The listing builds one solid part. Answer for the finished solid, in the listing's coordinates (mm). A direction names the side the tool comes from. Give positions to 0.01 mm unless a question says otherwise; leave off trailing zeros. Write each loop counter-clockwise with the first axis right and the second up, starting at its lowest first coordinate (ties: lowest second). Pieces come first, ordered by that corner, then holes. Notation, with made-up numbers: (78.25, -21) -> (89.25, -21) arc R25 ccw to (89.25, 17) -> close; hole circle Ø6 at (-3, -3). An arc over 180 degrees is marked (long way). Put each result on its own line as item: value. Start each with the question number.
1) For faces 1 (the flat face through (76.2, -8, 13)), 2 (the flat face through (-82.55, -8, 165)), 3 (the cylindrical face through (79.44, 20.35, 88.01)), determine the directions among +Z, -Z, +X, -X, +Y, -Y from which every point of the face is accessible in a straight line to the end or side of a thin tool.
2) Flat-ended cylindrical pins translate along their axes: pin 1 Ø2.5 at (y, z) = (-29.82, 158.75) entering from +X; pin 2 Ø1.9 at (x, y) = (-80, -18.5) entering from -Z; pin 3 Ø2 at (x, z) = (37, 61.5) entering from -Y; pin 4 Ø2 at (x, z) = (57.5, 140) entering from +Y. Find the tip coordinate at first contact, or state that the pin passes through.
3) A cutting plane is placed at C-C (x = 0). Write down the section's boundary in (y, z).
4) A cutting plane is placed at D-D (z = 92). Write down the section's boundary in (x, y) (3 decimals).
5) A cutting plane is placed at B-B (y = 80.5). Write down the section's boundary in (x, z).
6) A cutting plane is placed at A-A (y = -1.5). Write down the section's boundary in (x, z).
7) For a pull along X with two mould halves and no side action, classify faces 4 (the flat face through (-79, -39.977, 13)), 5 (the flat face through (-82.55, -8, 13)), 6 (the flat face through (-76.2, -8, 165)), 7 (the cylindrical face through (1.676, 99.704, 87.655)) as released by +X, released by -X, zero draft, split by the parting line, or undercut.
8) Find the intervals of material crossed by line 1 along X through (y, z) = (13.5, 159.5); line 2 along X through (y, z) = (84.5, 110); line 3 along Y through (x, z) = (-35, 93.5), in increasing order. Write a range as from..to.
from build123d import *

# Parameters (mm, degrees)
EXTRUDE_THIN1_DEPTH     = 177.8
SKETCH7_W               = 6.35
SKETCH7_H               = 25.4
BOSS_EXTRUDE2_DEPTH     = 63.5
SKETCH11_R              = 2
CUT_EXTRUDE1_DEPTH      = 6.35
MIRROR2_COPY_1_SKETCH_W = 6.35
MIRROR2_COPY_1_SKETCH_H = 25.4
MIRROR2_COPY_1_DEPTH    = 63.5
MIRROR2_COPY_2_SKETCH_R = 2
MIRROR2_COPY_2_DEPTH    = 6.35
BOSS_EXTRUDE3_DEPTH     = 127


with BuildPart() as part:
    # Sketch2 → Extrude-Thin1 (new body)
    with BuildSketch(Plane.XY):
        with BuildLine():
            ThreePointArc((76.2, 23.522786699), (0, 99.722786699), (-76.2, 23.522786699))
            Line((-76.2, 23.522786699), (-82.55, 23.522786699))
            ThreePointArc((-82.55, 23.522786699), (0, 106.072786699), (82.55, 23.522786699))
            Line((82.55, 23.522786699), (76.2, 23.522786699))
        make_face()
    extrude(amount=EXTRUDE_THIN1_DEPTH)

    # Sketch7 → Boss-Extrude2 (add)
    with BuildSketch(Plane.XZ.offset(-23.522786699)):
        with Locations((79.375, 12.7)):
            Rectangle(SKETCH7_W, SKETCH7_H)
    boss_extrude2 = extrude(amount=BOSS_EXTRUDE2_DEPTH)

    # Sketch11 → Cut-Extrude1 (cut)
    with BuildSketch(Plane.ZY.offset(-76.2)):
        with Locations((6.35, -29.817213301)):
            Circle(SKETCH11_R)
        with Locations((19.05, -29.817213301)):
            Circle(SKETCH11_R)
    cut_extrude1 = extrude(amount=-CUT_EXTRUDE1_DEPTH, mode=Mode.SUBTRACT)

    # Mirror1: Boss-Extrude2, Cut-Extrude1 across plane
    add(boss_extrude2.mirror(Plane.XY.offset(88.9)))
    add(cut_extrude1.mirror(Plane.XY.offset(88.9)), mode=Mode.SUBTRACT)

    # Mirror2: Boss-Extrude2, Cut-Extrude1 across plane
    add(boss_extrude2.mirror(Plane(origin=(0, 0, 0), x_dir=(0, 0, 1), z_dir=(1, 0, 0))))
    add(cut_extrude1.mirror(Plane(origin=(0, 0, 0), x_dir=(0, 0, 1), z_dir=(1, 0, 0))), mode=Mode.SUBTRACT)

    # Mirror2 copy 1 sketch → Mirror2 copy 1 (add)
    with BuildSketch(Plane(origin=(0, 23.522786699, 177.8), x_dir=(-1, 0, 0), z_dir=(0, -1, 0))):
        with Locations((79.375, 12.7)):
            Rectangle(MIRROR2_COPY_1_SKETCH_W, MIRROR2_COPY_1_SKETCH_H)
    extrude(amount=MIRROR2_COPY_1_DEPTH)

    # Mirror2 copy 2 sketch → Mirror2 copy 2 (cut)
    with BuildSketch(Plane(origin=(-76.2, 0, 177.8), x_dir=(0, 0, -1), z_dir=(1, 0, 0))):
        with Locations((6.35, -29.817213301)):
            Circle(MIRROR2_COPY_2_SKETCH_R)
        with Locations((19.05, -29.817213301)):
            Circle(MIRROR2_COPY_2_SKETCH_R)
    extrude(amount=-MIRROR2_COPY_2_DEPTH, mode=Mode.SUBTRACT)

    # Sketch15 → Boss-Extrude3 (add)
    with BuildSketch(Plane.XY.offset(25.4)):
        with BuildLine():
            Line((76.2, 23.522786699), (82.55, 23.522786699))
            ThreePointArc((82.55, 23.522786699), (79.375, 20.347786699), (76.2, 23.522786699))
        make_face()
    boss_extrude3 = extrude(amount=BOSS_EXTRUDE3_DEPTH)

    # Mirror3: Boss-Extrude3 across plane
    add(boss_extrude3.mirror(Plane(origin=(0, 0, 0), x_dir=(0, 0, 1), z_dir=(1, 0, 0))))


solid = part.part
Reply:
1. face 1: +Z, -Z, -Y
1. face 2: +Z, -Z, -X, +Y, -Y
1. face 3: -Y
2. pin 1: passes through
2. pin 2: stops at z = 0
2. pin 3: stops at y = 89.57
2. pin 4: stops at y = 83.71
3. outline: (99.72, 0) -> (106.07, 0) -> (106.07, 177.8) -> (99.72, 177.8) -> close
4. outline: (-82.55, 23.523) arc R3.175 ccw to (-76.2, 23.523) arc R76.2 cw to (76.2, 23.523) arc R3.175 ccw to (82.55, 23.523) arc R82.55 ccw to start
5. outline: (-59.73, 0) -> (-50.6, 0) -> (-50.6, 177.8) -> (-59.73, 177.8) -> close; (50.6, 0) -> (59.73, 0) -> (59.73, 177.8) -> (50.6, 177.8) -> close
6. outline: (-82.55, 0) -> (-76.2, 0) -> (-76.2, 25.4) -> (-82.55, 25.4) -> close; (-82.55, 152.4) -> (-76.2, 152.4) -> (-76.2, 177.8) -> (-82.55, 177.8) -> close; (76.2, 0) -> (82.55, 0) -> (82.55, 25.4) -> (76.2, 25.4) -> close; (76.2, 152.4) -> (82.55, 152.4) -> (82.55, 177.8) -> (76.2, 177.8) -> close
7. face 4: zero draft
7. face 5: released by -X
7. face 6: undercut
7. face 7: undercut
8. line 1: x = -82.55..-76.2, 76.2..82.55
8. line 2: x = -55.64..-45.7, 45.7..55.64
8. line 3: y = 91.21..98.29
